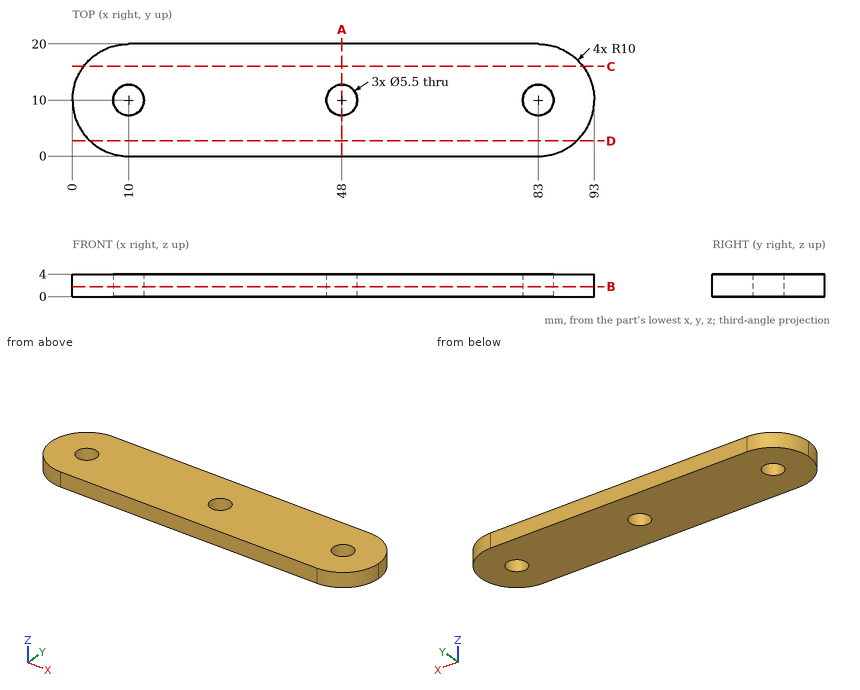
Input: dimensioned drawing with shaded views. Units: mm. Origin: part minimum x, y, z. Coordinates: 2 decimals unless noted, no trailing zeros. Write each loop counter-clockwise with the first axis right and the second up, starting at its lowest first coordinate (ties: lowest second). Pieces come first, ordered by that corner, then holes. Notation, with made-up numbers: M 5,24.5 L 64,24.5 A21 cw 64,62.5 Z; hole C 47,59.25 d11. An arc over 180 degrees is marked long. Use one line per item in the form item = value.
Q1. Section A-A (x = 48). Return loops of the section in (y, z), plus the area to 3 significant figures.
Answer below:
outline = M 0,0 L 7.25,0 L 7.25,4 L 0,4 Z; M 12.75,0 L 20,0 L 20,4 L 12.75,4 Z
area = 58.0 mm²
Q2. Section C-C (y = 16). Return loops of the section in (x, z), plus the area to 3 significant figures.
Answer below:
outline = M 2,0 L 91,0 L 91,4 L 2,4 Z
area = 356 mm²
Q3. First-contact query: pin 1 (1 mm diameter, centred on y = 17.5, z = 3.5, fed in from -X). Flat tip, straight axial feed; report the tip coordinate or a pass-through.
Answer below:
pin_1 = 2.86
Q4. Section B-B (z = 1.8). Count the separate pieces of the cut face and the enclosed holes in it, plus the area to 3 significant figures.
Answer below:
separate_pieces = 1
enclosed_holes = 3
area = 1,700 mm²
Q5. Material intervals for probe 1 along X at (y, z) = (10, 2.3); probe 2 along Y at (x, z) = (10, 1.65); probe 3 along X at (y, z) = (9.25, 0.95), sorted ascending. Write a range as from..to.
Answer below:
probe_1 = 0..7.25, 12.75..45.25, 50.75..80.25, 85.75..93
probe_2 = 0..7.25, 12.75..20
probe_3 = 0.03..7.35, 12.65..45.35, 50.65..80.35, 85.65..92.97
Q6. Section D-D (y = 2.75). Return loops of the section in (x, z).
Answer below:
outline = M 3.11,0 L 89.89,0 L 89.89,4 L 3.11,4 Z
